Can you work these out from the model? Positions are in its coordinate system, mm. Face numbers are marked on the shaded views. A direction names the side the tool comes from. Give positions to 0.01 mm unless a question says otherwise; leave off trailing zeros. Write each loop counter-clockwise with the first axis right and the second up, starting at its lowest first coordinate (ties: lowest second). Pieces come first, ordered by that corner, then holes.
```python
from build123d import *

# Parameters (mm, degrees)
F2_SIZE = 0.762
F3_R    = 0.254


with BuildPart() as f1:
    # F0 (on Right) → F1 (revolve)
    with BuildSketch(Plane.YZ):
        Polygon((-18.7706, 15.1765), (0, 15.1765), (18.7706, 15.1765), (18.7706, 20.9804), (31.4706, 20.9804), (31.4706, 49.3522), (6.7945, 49.3522), (6.7945, 44.8818), (1.7145, 44.8818), (1.7145, 32.1818), (-1.7145, 32.1818), (-1.7145, 44.8818), (-6.7945, 44.8818), (-6.7945, 49.3522), (-31.4706, 49.3522), (-31.4706, 20.9804), (-18.7706, 20.9804), align=None)
    revolve(axis=Axis((0, -0.984378, 0), (0, 1, 0)))

    # F2
    f2_edges = [f1.edges().sort_by_distance(p)[0] for p in [
        (0, 1.7145, -44.8818),
        (0, -1.7145, -44.8818),
    ]]
    chamfer(f2_edges, length=F2_SIZE)

    # F3
    f3_edges = [f1.edges().sort_by_distance(p)[0] for p in [
        (0, -1.7145, -32.1818),
        (0, 1.7145, -32.1818),
    ]]
    fillet(f3_edges, radius=F3_R)


solid = f1.part
```
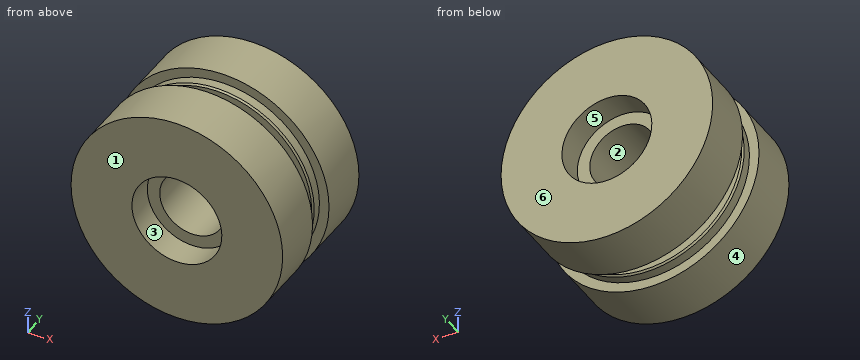
1) If we mould it in two halves opening along X, with no side actions, what happens to the marked faces 1, 2, 3 and 4? For each: +X half, -X half, draft (parallel to the pull), parting line (faces both ways), or undercut.
Values follow:
face 1: draft
face 2: undercut
face 3: undercut
face 4: parting line
2) For pin 1 Ø12.5 at (x, z) = (9.5, -2.5) entering from -Y; pin 2 Ø2 at (y, z) = (11.5, -22.5) entering from +X; pin 3 Ø5 at (y, z) = (3, 18.5) entering from -X, each with a flat end and sliding along its axis, tell me the tip position at first contact or that it passes through.
Values follow:
pin 1: stops at y = -18.77
pin 2: stops at x = 44.42
pin 3: stops at x = -41.93
3) For the marked faces 5 and 6, which set-ups out of +Z, -Z, +X, -X, +Y, -Y let a thin tool reach every point of the face, with its end or its side?
Values follow:
face 5: +Y
face 6: +Z, -Z, +X, -X, +Y
4) Suppose I cut it at B-B on y = -21. Write out the boundary of the cut face in (x, z), plus the area to 3 significant figures.
Values follow:
outline: circle Ø98.7 at (0, 0); hole circle Ø41.96 at (0, 0)
area: 6,270 mm2
5) Please list where these lines run through material, in increasing order: L1, parallel to X at y = 11, z = 0; L2, parallel to Y at x = 25, z = -24; L3, parallel to X at y = 21.5, z = 0.
Values follow:
L1: x = -49.35 to -15.18, 15.18 to 49.35
L2: y = -31.47 to -1.71, 1.71 to 31.47
L3: x = -49.35 to -20.98, 20.98 to 49.35
6) Suppose I cut it at A-A on y = 11. Write out the boundary of the cut face in (x, z), plus the area to 3 significant figures.
Values follow:
outline: circle Ø98.7 at (0, 0); hole circle Ø30.35 at (0, 0)
area: 6,930 mm2
